```python
from build123d import *

# Parameters (mm, degrees)
BOSS_EXTRUDE1_DEPTH = 50
SKETCH3_R           = 105
CUT_EXTRUDE1_DEPTH  = 50
SKETCH4_R           = 15
CUT_EXTRUDE3_DEPTH  = 50
SKETCH7_R           = 30
CUT_EXTRUDE4_DEPTH  = 10


with BuildPart() as part:
    # Sketch2 → Boss-Extrude1 (new body)
    with BuildSketch(Plane.XY):
        with BuildLine():
            Line((-160, 180), (160, 180))
            ThreePointArc((160, 180), (174.142135624, 174.142135624), (180, 160))
            Line((180, 160), (180, -160))
            ThreePointArc((180, -160), (174.142135624, -174.142135624), (160, -180))
            Line((160, -180), (-160, -180))
            ThreePointArc((-160, -180), (-174.142135624, -174.142135624), (-180, -160))
            Line((-180, -160), (-180, 160))
            ThreePointArc((-180, 160), (-174.142135624, 174.142135624), (-160, 180))
        make_face()
    extrude(amount=BOSS_EXTRUDE1_DEPTH)

    # Sketch3 → Cut-Extrude1 (cut)
    with BuildSketch(Plane.XY.offset(50)):
        Circle(SKETCH3_R)
    extrude(amount=-CUT_EXTRUDE1_DEPTH, mode=Mode.SUBTRACT)

    # Sketch4 → Cut-Extrude3 (cut)
    with BuildSketch(Plane.XY.offset(50)):
        with Locations((-130, 130)):
            Circle(SKETCH4_R)
        with Locations((-130, -130)):
            Circle(SKETCH4_R)
        with Locations((130, -130)):
            Circle(SKETCH4_R)
        with Locations((130, 130)):
            Circle(SKETCH4_R)
    extrude(amount=-CUT_EXTRUDE3_DEPTH, mode=Mode.SUBTRACT)

    # Sketch7 → Cut-Extrude4 (cut)
    with BuildSketch(Plane.XY.offset(50)):
        with Locations((-130, 130)):
            Circle(SKETCH7_R)
        with Locations((130, 130)):
            Circle(SKETCH7_R)
        with Locations((130, -130)):
            Circle(SKETCH7_R)
        with Locations((-130, -130)):
            Circle(SKETCH7_R)
    extrude(amount=-CUT_EXTRUDE4_DEPTH, mode=Mode.SUBTRACT)


solid = part.part
```
Geometry check sheet. Reference: the model listing, model coordinates, mm. A direction names the side the tool comes from. Round coordinates to 2 decimals unless told otherwise and drop trailing zeros. Loops run counter-clockwise (first coordinate to the right, second up) from the corner with the lowest first, then second, coordinate; pieces in that order, holes last. Notation, with made-up numbers: (14.25, 23.5) - (47.25, 23.5) arc R29 ccw to (47.25, 45.5) - close; hole circle Ø5 at (27.25, 50). An arc over 180 degrees is marked (long way). Write item = value, one per line. Start each with the question number.
1. Section check C-C on z = 25.5. Enter the section's corners in (x, y), then the cut area to 3 significant figures.
2. Depth check by flat-ended pin: pin 1 (18 mm diameter, centred on x = -130, y = 130, fed in from -Z). Enter the tip coordinate at first touch or a pass-through.
3. Mould release check, pull along X, two halves, no side actions. Record for faces 1 (the face through (174.297, -173.986, 24.65)), 2 (the face through (-174.297, 173.986, 24.65)), 3 (the face through (123.497, -159.287, 45.07)): released by +X, released by -X, zero draft, split by the parting line, or undercut.
4. Thickness scan on line 1 (Y direction, x = 130, z = 44.25); line 2 (Y direction, x = -130, z = 19); line 3 (X direction, y = -23, z = 21). Record the ranges inside material, lowest first.
5. Section check B-B on x = 130. Enter the section's corners in (y, z).
6. Section check A-A on y = 0. Enter the section's corners in (x, z).
7. Set-up check for faces 4 (the face through (-136.503, -159.287, 45.07)), 5 (the face through (-173.986, -174.297, 24.65)): record each of +Z, -Z, +X, -X, +Y, -Y from which the full face is reachable in a straight line by a thin tool's end or side.
Working result:
q1.outline = (-180, -160) arc R20 ccw to (-160, -180) - (160, -180) arc R20 ccw to (180, -160) - (180, 160) arc R20 ccw to (160, 180) - (-160, 180) arc R20 ccw to (-180, 160) - close; hole circle Ø30 at (-130, -130); hole circle Ø30 at (-130, 130); hole circle Ø210 at (0, 0); hole circle Ø30 at (130, -130); hole circle Ø30 at (130, 130)
q1.area = 91,800 mm^2
q2.pin_1 = through
q3.face_1 = released by +X
q3.face_2 = released by -X
q3.face_3 = undercut
q4.line_1 = -180 to -160, -100 to 100, 160 to 180
q4.line_2 = -180 to -145, -115 to 115, 145 to 180
q4.line_3 = -180 to -102.45, 102.45 to 180
q5.outline = (-180, 0) - (-145, 0) - (-145, 40) - (-160, 40) - (-160, 50) - (-180, 50) - close; (-115, 0) - (115, 0) - (115, 40) - (100, 40) - (100, 50) - (-100, 50) - (-100, 40) - (-115, 40) - close; (145, 0) - (180, 0) - (180, 50) - (160, 50) - (160, 40) - (145, 40) - close
q6.outline = (-180, 0) - (-105, 0) - (-105, 50) - (-180, 50) - close; (105, 0) - (180, 0) - (180, 50) - (105, 50) - close
q7.face_4 = +Z
q7.face_5 = +Z, -Z, -X, -Y
